```python
from build123d import *

# Parameters (mm, degrees)
BOSS_EXTRUDE1_DEPTH      = 3
BOSS_EXTRUDE1_DEPTH_BACK = 3
SKETCH1_W                = 90
SKETCH1_H                = 64
SKETCH1_4_W              = 104
SKETCH1_4_H              = 74
SKETCH1_4_W_2            = 90
SKETCH1_4_H_2            = 64
BOSS_EXTRUDE3_DEPTH      = 3
CUT_EXTRUDE1_DEPTH       = 120.18892566
CUT_EXTRUDE1_DEPTH_BACK  = 120.18892566
SKETCH2_W                = 60
SKETCH2_H                = 10
SKETCH3_W                = 5
SKETCH3_H                = 41
CUT_EXTRUDE2_DEPTH       = 120.18892566


with BuildPart() as part:
    # Sketch1 → Boss-Extrude1 (new, two sides: drawn at the far end of the back side and taken through both)
    with BuildSketch(Plane(origin=(0, 0, 0), x_dir=(1, 0, 0), z_dir=(0, 1, 0)).offset(-BOSS_EXTRUDE1_DEPTH_BACK)):
        with Locations((45, 32)):
            Rectangle(SKETCH1_W, SKETCH1_H)
    extrude(amount=BOSS_EXTRUDE1_DEPTH + BOSS_EXTRUDE1_DEPTH_BACK)

    # Sketch1<4> → Boss-Extrude3 (add)
    with BuildSketch(Plane(origin=(0, 0, 0), x_dir=(1, 0, 0), z_dir=(0, 1, 0))):
        with Locations((45, 32)):
            Rectangle(SKETCH1_4_W, SKETCH1_4_H)
        with Locations((45, 32)):
            Rectangle(SKETCH1_4_W_2, SKETCH1_4_H_2, mode=Mode.SUBTRACT)
    extrude(amount=BOSS_EXTRUDE3_DEPTH)

    # Sketch2 → Cut-Extrude1 (cut, two sides: drawn at the far end of the back side and taken through both)
    with BuildSketch(Plane.XZ.offset(3).offset(-CUT_EXTRUDE1_DEPTH_BACK)):
        with Locations((60, -5)):
            Rectangle(SKETCH2_W, SKETCH2_H)
    extrude(amount=CUT_EXTRUDE1_DEPTH + CUT_EXTRUDE1_DEPTH_BACK, mode=Mode.SUBTRACT)

    # Sketch3 → Cut-Extrude2 (cut, through all)
    with BuildSketch(Plane(origin=(0, 3, 0), x_dir=(1, 0, 0), z_dir=(0, 1, 0))):
        with Locations((37.5, 38.5)):
            Rectangle(SKETCH3_W, SKETCH3_H)
        with Locations((52.5, 38.5)):
            Rectangle(SKETCH3_W, SKETCH3_H)
        with Locations((82.5, 38.5)):
            Rectangle(SKETCH3_W, SKETCH3_H)
        with Locations((67.5, 38.5)):
            Rectangle(SKETCH3_W, SKETCH3_H)
    extrude(amount=-CUT_EXTRUDE2_DEPTH, mode=Mode.SUBTRACT)


solid = part.part
```
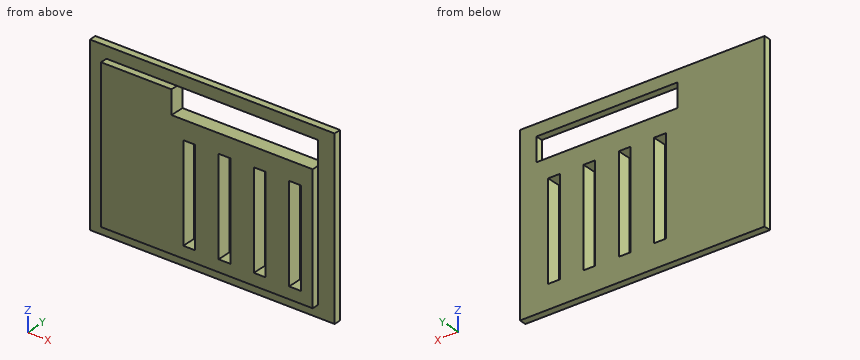
Can you work these out from the model? Positions are in its coordinate system, mm. Give positions to 0.01 mm unless a question says otherwise; leave off trailing zeros. Write each loop counter-clockwise with the first axis right and the second up, starting at its lowest first coordinate (ties: lowest second). Pieces come first, ordered by that corner, then holes. Notation, with made-up numbers: (-14.5, -15) -> (31.5, -15) arc R21 cw to (31.5, 23) -> close; hole circle Ø5 at (65, 66). An arc over 180 degrees is marked (long way). One line per item, written item: value.
Q1. Imagine slicing it at A-A on x = 38. Please give me the cut outline in (y, z).
Results found:
outline: (-3, -64) -> (0, -64) -> (0, -69) -> (3, -69) -> (3, -59) -> (-3, -59) -> close; (-3, -18) -> (3, -18) -> (3, -10) -> (-3, -10) -> close; (0, 0) -> (3, 0) -> (3, 5) -> (0, 5) -> close
Q2. For P1, Ø1.5, axis at x = 67.5, y = -1, coming from the +Z side, with a flat end and sliding along its axis, tell me the tip position at first contact or that it passes through.
Results found:
P1: stops at z = -10
Q3. Please list where these lines run through material, in increasing order: line 1 (X direction, y = 1.7, z = -40.5); line 2 (Z direction, x = 81, y = 2.35); line 3 (X direction, y = -1.1, z = -44). Write a range as [from, to].
Results found:
line 1: x = [-7, 35], [40, 50], [55, 65], [70, 80], [85, 97]
line 2: z = [-69, -59], [-18, -10], [0, 5]
line 3: x = [0, 35], [40, 50], [55, 65], [70, 80], [85, 90]
Q4. Imagine slicing it at D-D on y = 1.9. Please give me the cut outline in (x, z), and give its area (3 significant figures).
Results found:
outline: (-7, -69) -> (97, -69) -> (97, 5) -> (-7, 5) -> close; hole (30, -10) -> (90, -10) -> (90, 0) -> (30, 0) -> close; hole (35, -59) -> (40, -59) -> (40, -18) -> (35, -18) -> close; hole (50, -59) -> (55, -59) -> (55, -18) -> (50, -18) -> close; hole (65, -59) -> (70, -59) -> (70, -18) -> (65, -18) -> close; hole (80, -59) -> (85, -59) -> (85, -18) -> (80, -18) -> close
area: 6,280 mm^2
Q5. Imagine slicing it at B-B on z = -5. Please give me the cut outline in (x, y), and give its area (3 significant figures).
Results found:
outline: (-7, 0) -> (0, 0) -> (0, -3) -> (30, -3) -> (30, 3) -> (-7, 3) -> close; (90, 0) -> (97, 0) -> (97, 3) -> (90, 3) -> close
area: 222 mm^2
Q6. Imagine slicing it at C-C on z = -49. Please give me the cut outline in (x, y), and give its area (3 significant figures).
Results found:
outline: (-7, 0) -> (0, 0) -> (0, -3) -> (35, -3) -> (35, 3) -> (-7, 3) -> close; (40, -3) -> (50, -3) -> (50, 3) -> (40, 3) -> close; (55, -3) -> (65, -3) -> (65, 3) -> (55, 3) -> close; (70, -3) -> (80, -3) -> (80, 3) -> (70, 3) -> close; (85, -3) -> (90, -3) -> (90, 0) -> (97, 0) -> (97, 3) -> (85, 3) -> close
area: 462 mm^2
